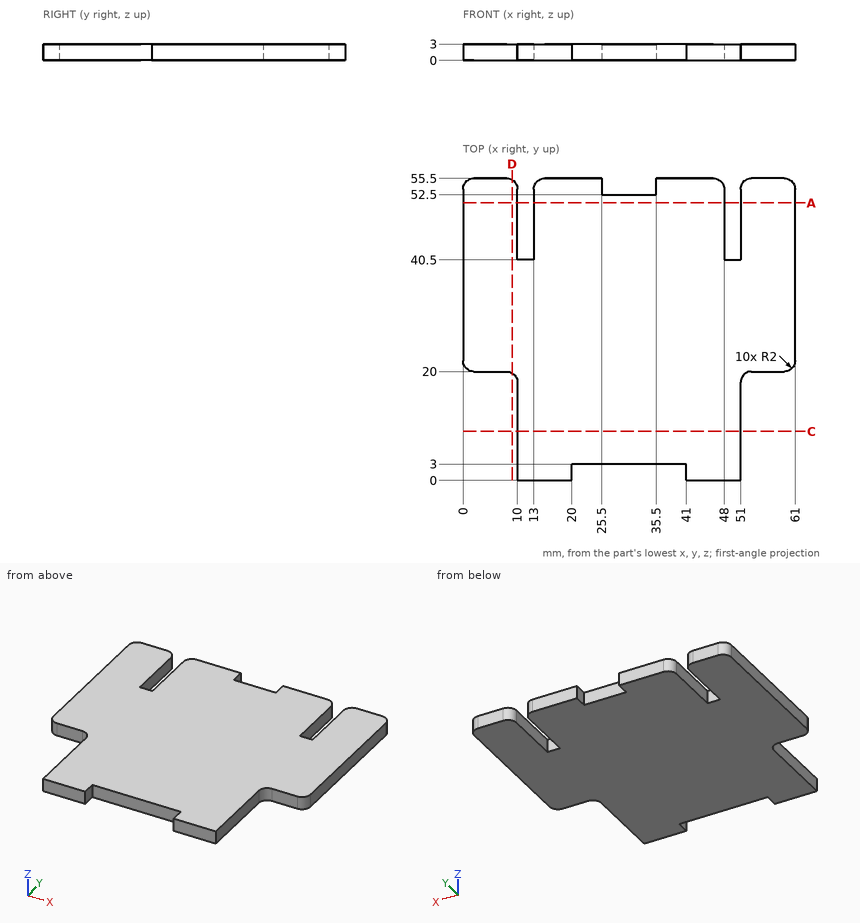
Design review of the part shown in the three views and the two pictorial views. Dimensions are in mm from the part's minimum x, y and z. Give positions to 0.01 mm unless a question says otherwise; leave off trailing zeros. Loops run counter-clockwise (first coordinate to the right, second up) from the corner with the lowest first, then second, coordinate; pieces in that order, holes last. Notation, with made-up numbers: (-33.75, 26) -> (-12.75, 26) arc R28 ccw to (-12.75, 47) -> close; hole circle Ø9 at (51.25, 65.25). An arc over 180 degrees is marked (long way). Answer as a JSON object with one key per item and string values. Group by question number.
Q1. Take a section at D-D (x = 9). Write out the cut boundary in (y, z), plus the area to 4 significant figures.
Q2. Take a section at C-C (y = 9). Write out the cut boundary in (x, z), plus the area to 3 significant figures.
Q3. Insertion check: pin 1 (1.5 mm diameter, centred on x = 31, z = 2, fed in from +Y); pin 2 (0.9 mm diameter, centred on y = 5.5, z = 1, fed in from -X); pin 3 (0.9 mm diameter, centred on x = 55, z = 1, fed in from -Y). Each pin has a flat end and moves straight along its axis. Give the tip position at first contact, or say it passes through.
Q4. Wall thickness on line 1 along X through (y, z) = (50, 1.1); line 2 along Y through (x, z) = (6, 2.7); line 3 along X through (y, z) = (15.5, 2.05): over which ranges is each line inside the solid? List them lowest first.
Q5. Take a section at A-A (y = 51). Write out the cut boundary in (x, z), plus the area to 3 significant figures.
Answer below:
{
 "1": {"outline": "(19.73, 0) -> (55.23, 0) -> (55.23, 3) -> (19.73, 3) -> close", "area": "106.5 mm2"},
 "2": {"outline": "(10, 0) -> (51, 0) -> (51, 3) -> (10, 3) -> close", "area": "123 mm2"},
 "3": {"pin 1": "stops at y = 52.5", "pin 2": "stops at x = 10", "pin 3": "stops at y = 20"},
 "4": {"line 1": "x = 0 to 10, 13 to 48, 51 to 61", "line 2": "y = 20 to 55.5", "line 3": "x = 10 to 51"},
 "5": {"outline": "(0, 0) -> (10, 0) -> (10, 3) -> (0, 3) -> close; (13, 0) -> (48, 0) -> (48, 3) -> (13, 3) -> close; (51, 0) -> (61, 0) -> (61, 3) -> (51, 3) -> close", "area": "165 mm2"}
}
